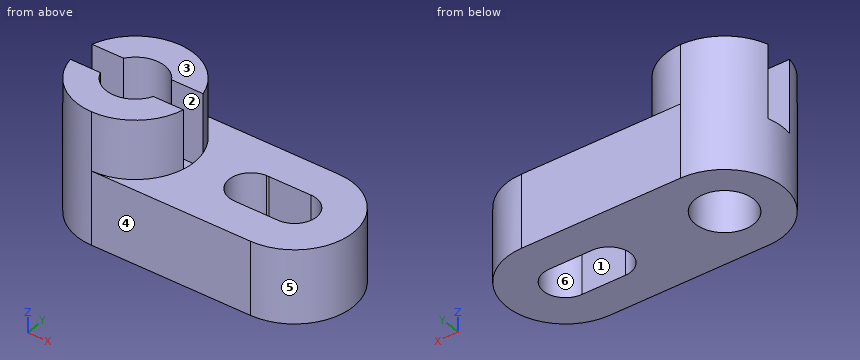
```python
from build123d import *

# Parameters (mm, degrees)
F1_DEPTH = 25
F3_DEPTH = 20
F4_R     = 10
F5_DEPTH = 77.8
F7_DEPTH = 25
F9_DEPTH = 25


# Not quite as in the source:
# - ends of sketch curves that miss each other by under 0.0002 mm in the source are joined


with BuildPart() as f1:
    # F0 (on Top) → F1 (new body)
    with BuildSketch(Plane.XY):
        with BuildLine():
            Line((55, 20), (0, 20))
            ThreePointArc((0, 20), (-20, 0), (0, -20))
            Line((0, -20), (55, -20))
            ThreePointArc((55, -20), (75, 0), (55, 20))
        make_face()
    extrude(amount=F1_DEPTH)

    # F2 (on face) → F3 (join)
    with BuildSketch(Plane.XY.offset(25)):
        with BuildLine():
            ThreePointArc((0, -20), (14.1421356237, -14.1421356237), (20, 0))
            ThreePointArc((20, 0), (14.1421356237, 14.1421356237), (0, 20))
            ThreePointArc((0, 20), (-20, 0), (0, -20))
        make_face()
    extrude(amount=F3_DEPTH)

    # F4 (on face) → F5 (cut)
    with BuildSketch(Plane.XY.offset(45)):
        Circle(F4_R)
    extrude(amount=-F5_DEPTH, mode=Mode.SUBTRACT)

    # F6 (on face) → F7 (cut)
    with BuildSketch(Plane.XY.offset(45)):
        with BuildLine():
            ThreePointArc((-9.2726967228, -3.7439411704), (-9.9478279478, 1.02015642), (-8.3197954675, 5.5480630295))
            Line((-8.3197954675, 5.5480630295), (-19.2150721212, 5.5480630295))
            ThreePointArc((-19.2150721212, 5.5480630295), (-19.9784825468, 0.9274886135), (-19.6464476309, -3.7439411704))
            Line((-19.6464476309, -3.7439411704), (-9.2726967228, -3.7439411704))
        make_face()
        with BuildLine():
            Line((19.2537545525, 5.4122948584), (8.4087492748, 5.4122948584))
            ThreePointArc((8.4087492748, 5.4122948584), (9.593943213, 2.8206831843), (10, 0))
            ThreePointArc((10, 0), (9.7948219983, -2.0153069299), (9.1877075957, -3.94791453))
            Line((9.1877075957, -3.94791453), (19.6064777781, -3.94791453))
            ThreePointArc((19.6064777781, -3.94791453), (19.9013762786, -1.9837394534), (20, 0))
            ThreePointArc((20, 0), (19.8125602971, 2.7317493435), (19.2537545525, 5.4122948584))
        make_face()
    extrude(amount=-F7_DEPTH, mode=Mode.SUBTRACT)

    # F8 (on face) → F9 (cut)
    with BuildSketch(Plane.XY.offset(25)):
        with BuildLine():
            Line((54.9931789181, 7.4999968982), (40.4453485752, 7.4867659671))
            Line((40.4453485752, 7.4867659671), (39.5410340755, 7.485943513))
            ThreePointArc((39.5410340755, 7.485943513), (32.5035149454, -0.229590562), (40, -7.5))
            Line((40, -7.5), (55, -7.5))
            ThreePointArc((55, -7.5), (62.4999992241, 0.0034115228), (54.9931789181, 7.4999968982))
        make_face()
    extrude(amount=-F9_DEPTH, mode=Mode.SUBTRACT)


solid = f1.part
```
Design review of the part built by this model. Coordinates are the model's own, in mm. Face numbers are marked on the shaded views. A direction names the side the tool comes from. Coordinates: 2 decimals unless noted, no trailing zeros. Loops run counter-clockwise (first coordinate to the right, second up) from the corner with the lowest first, then second, coordinate; pieces in that order, holes last. Notation, with made-up numbers: M 35.5,-3 L 54.5,-3 A18 ccw 54.5,12 Z; hole C 51,50 d6. An arc over 180 degrees is marked long. One line per question, with ' | ' between items.
(1) Wall thickness on probe 1 along X at (y, z) = (0, 16.5); probe 2 along Y at (x, z) = (48, 6.5); probe 3 along Y at (x, z) = (0, 22): over which ranges is each line inside the solid? List them lowest first.
Filled in:
probe 1: x = -20 to -10, 10 to 32.5, 62.5 to 75 | probe 2: y = -20 to -7.5, 7.49 to 20 | probe 3: y = -20 to -10, 10 to 20
(2) We need section A-A (z = 42). Give the boundary of the cut face in (x, y), and give its area (3 significant figures).
Filled in:
outline: M -19.65,-3.74 A20 ccw 19.61,-3.95 L 9.19,-3.95 A10 cw -9.27,-3.74 Z; M -19.22,5.55 L -8.32,5.55 A10 cw 8.41,5.41 L 19.25,5.41 A20 ccw Z | area: 752 mm^2
(3) We need section B-B (z = 14). Give the boundary of the cut face in (x, y).
Filled in:
outline: M 0,-20 L 55,-20 A20 ccw 55,20 L 0,20 A20 ccw Z; hole C 0,0 d20; hole M 39.54,7.49 A7.5 ccw 40,-7.5 L 55,-7.5 A7.5 ccw 54.99,7.5 Z
(4) We need section D-D (y = -1). Give the boundary of the cut face in (x, z), and give its area (3 significant figures).
Filled in:
outline: M -19.97,0 L -9.95,0 L -9.95,20 L -19.97,20 Z; M 9.95,0 L 32.57,0 L 32.57,25 L 19.97,25 L 19.97,20 L 9.95,20 Z; M 62.43,0 L 74.97,0 L 74.97,25 L 62.43,25 Z | area: 1,030 mm^2
(5) Machinability: for the marked faces 1, 2 and 3, which of the approach directions +Z, -Z, +X, -X, +Y, -Y give a long, thin tool a straight path to every point of the face, cutting with its end or side? Answer none if there is none.
Filled in:
face 1: +Z, -Z | face 2: +Z, -X | face 3: +Z, +X, -X, +Y, -Y
(6) Draft analysis for pull direction X (two halves, no side actions). For the marked faces 4, 5 and 6, state which applies: released by +X, released by -X, zero draft, split by the parting line, or undercut.
Filled in:
face 4: zero draft | face 5: released by +X | face 6: undercut
(7) We need section C-C (x = 37). Give the boundary of the cut face in (y, z), and give its area (3 significant figures).
Filled in:
outline: M -20,0 L -6.87,0 L -6.87,25 L -20,25 Z; M 6.87,0 L 20,0 L 20,25 L 6.87,25 Z | area: 656 mm^2
(8) For pin 1 Ø8.5 at (x, z) = (15.5, 36.5) entering from +Y; pin 2 Ø3 at (x, y) = (13.5, -1.5) entering from +Z; pin 3 Ø5.5 at (x, z) = (12, 29) entering from -Y; pin 4 Ø2 at (x, y) = (-4.5, -15) entering from -Z, all flat-tipped, find the tip position at first contact; note any pin that passes through.
Filled in:
pin 1: stops at y = 16.54 | pin 2: stops at z = 20 | pin 3: stops at y = -17.73 | pin 4: stops at z = 0
